Build history of the part. All positions in model axes, mm. A direction names the side the tool comes from. Round coordinates to 2 decimals unless told otherwise and drop trailing zeros. Write each loop counter-clockwise with the first axis right and the second up, starting at its lowest first coordinate (ties: lowest second). Pieces come first, ordered by that corner, then holes.
Autodesk Inventor part; units mm, degrees
ref_plane "YZ Plane" through (0, 0, 0) normal (1, 0, 0) x (0, 1, 0)
ref_plane "XZ Plane" through (0, 0, 0) normal (0, 1, 0) x (-1, 0, 0)
ref_plane "XY Plane" through (0, 0, 0) normal (0, 0, 1) x (1, 0, 0)
sketch "Sketch2" plane through (0, 0, 0) normal (0, 0, 1) x (1, 0, 0)
  line L0 (-10.8368, 23.5104) -> (-10.8368, -29.6906) construction
  line L1 (-37.8996, -2.6413) -> (16.2259, -2.6413) construction
  circle A0 centre (-28.9216, 37.4694) radius 2.4892
  circle A1 centre (7.248, 37.4694) radius 2.4892
  circle A2 centre (-28.9216, -20.4172) radius 2.4892
  circle A3 centre (7.248, -20.4172) radius 2.4892
  line L2 (-28.9216, 37.4694) -> (7.248, 37.4694) construction
  line L3 (7.248, 37.4694) -> (7.248, -20.4172) construction
  line L4 (7.248, -20.4172) -> (-28.9216, -20.4172) construction
  line L5 (-28.9216, -20.4172) -> (-28.9216, 37.4694) construction
  line L6 (-41.3549, 42.4478) -> (19.6813, 42.4478)
  line L7 (19.6813, 42.4478) -> (19.6813, -24.2272)
  line L8 (19.6813, -24.2272) -> (-41.3549, -24.2272)
  line L9 (-41.3549, -24.2272) -> (-41.3549, 42.4478)
  line L10 (-10.8368, 42.4478) -> (-10.8368, -24.2272) construction
  point P0 (0, 0)
  point P1 (-10.8368, -2.6413)
  dimension "d9" = 36.1696
  dimension "d10" = 57.8866
  dimension "d11" = 4.9784
  dimension "d12" = 61.0362
  dimension "d13" = 66.675
  dimension "d15" = 3.81
extrude "Extrusion1" add sketch "Sketch2" along normal blind 9.525
sketch "Sketch3" plane through (0, 0, 9.525) normal (0, 0, 1) x (1, 0, 0)
  line L0 (-41.3549, 34.1928) -> (19.6813, 34.1928)
  line L1 (19.6813, 34.1928) -> (19.6813, -16.6072)
  line L2 (19.6813, -16.6072) -> (-41.3549, -16.6072)
  line L3 (-41.3549, -16.6072) -> (-41.3549, 34.1928)
  line L4 (19.6813, -24.2272) -> (19.6813, 42.4478)
  line L5 (-41.3549, 42.4478) -> (-41.3549, -24.2272)
  line L6 (-41.3549, -24.2272) -> (19.6813, -24.2272)
  point P0 (0, 0)
  dimension "d18" = 50.8
  dimension "d20" = 7.62
extrude "Extrusion2" cut sketch "Sketch3" against normal blind 4.7498 contours L0 L1 L2 L3
chamfer "Chamfer1" distance 9.525 angle 45 4 edges at (19.6813, 42.4478, 4.7625) (-41.3549, 42.4478, 4.7625) (-41.3549, -24.2272, 4.7625) (19.6813, -24.2272, 4.7625)
fillet "Fillet1" radius 2.54 4 edges at (18.4113, 34.1928, 7.1501) (17.7763, -16.6072, 7.1501) (-39.4499, -16.6072, 7.1501) (-40.0849, 34.1928, 7.1501)
sketch "Sketch4" plane through (0, 0, 4.7752) normal (0, 0, 1) x (1, 0, 0)
  circle A0 centre (-10.8368, 7.2053) radius 14.2748
  line L0 (-41.3549, -14.7022) -> (-41.3549, 32.9228)
  line L1 (11.6442, -16.6072) -> (-33.3178, -16.6072)
  point P0 (0, 0)
  dimension "d27" = 30.5181
  dimension "d28" = 23.8125
  dimension "d29" = 28.5496
extrude "Extrusion3" cut sketch "Sketch4" against normal blind 4.7752
sketch "Sketch5" plane through (0, 0, 4.7752) normal (0, 0, 1) x (1, 0, 0)
  circle A0 centre (-10.8368, 7.2053) radius 14.2748
  circle A1 centre (-10.8368, 7.2053) radius 15.9766
  point P0 (0, 0)
  dimension "d32" = 31.9532
extrude "Extrusion4" cut sketch "Sketch5" against normal blind 1.6002
sketch "Sketch6" plane through (0, 0, 4.7752) normal (0, 0, 1) x (1, 0, 0)
  circle A0 centre (-10.8368, 7.2053) radius 14.2748
  circle A1 centre (-10.8368, 7.2053) radius 14.2748
  circle A2 centre (-10.8368, 7.2053) radius 23.8125 construction
  circle A3 centre (-34.6493, 7.2053) radius 2.4892
  point P0 (0, 0)
  dimension "d35" = 47.625
  dimension "d36" = 4.9784
extrude "Extrusion5" cut sketch "Sketch6" against normal through all contours A3
pattern_circular "Circular Pattern1" count 6 over 360 about axis through (-10.8368, 7.2053, 4.7752) along (0, 0, -1) of "Extrusion5"
sketch "Sketch7" plane through (0, 0, 4.7752) normal (0, 0, 1) x (1, 0, 0)
  circle A0 centre (-10.8368, 7.2053) radius 14.2748
  arc A1 (-5.4756, 27.2137) -> (-16.1981, 27.2137) centre (-10.8368, 7.2053) ccw
  arc A2 (-4.1608, 32.1206) -> (-17.5129, 32.1206) centre (-10.8368, 7.2053) ccw
  line L0 (-10.8368, 7.2053) -> (-10.8368, 32.9995) construction
  line L1 (-16.1981, 27.2137) -> (-17.5129, 32.1206)
  line L2 (-5.4756, 27.2137) -> (-4.1608, 32.1206)
  point P0 (0, 0)
  dimension "d42" = 5.08
extrude "Extrusion6" cut sketch "Sketch7" against normal through all contours A1 L1 A2 L2
pattern_circular "Circular Pattern2" count 6 over 360 about axis through (-10.8368, 7.2053, 4.7752) along (0, 0, -1) of "Extrusion6"
sketch "Sketch8" plane through (0, 0, 9.525) normal (0, 0, 1) x (1, 0, 0)
  line L0 (10.1563, 42.4478) -> (-31.8299, 42.4478)
  arc A0 (-25.4799, 42.4478) -> (3.8063, 42.4478) centre (-10.8368, 63.2021) ccw
  point P0 (0, 0)
  dimension "d49" = 6.35
  dimension "d50" = 6.35
  dimension "d51" = 25.4
extrude "Extrusion7" cut sketch "Sketch8" against normal through all
fillet "Fillet2" radius 2.54 2 edges at (-25.4799, 42.4478, 4.7625) (3.8063, 42.4478, 4.7625)
equation "\"d15\" = d14"
equation "\"d20\" = d19"
equation "\"d14\" = 3.81"
equation "\"d19\" = 2 * d14"
properties part number "Versa Chassis Bearing Block"
1) Wall check: L1, parallel to X at y = 7, z = 0.5; L2, parallel to X at y = -19, z = 7.75; L3, parallel to X at y = 14.5, z = 4.25. Give the ranges that are in metal, low to high.
Results:
L1: x = -41.35 to -37.13, -32.17 to -25.11, 3.44 to 10.49, 15.46 to 19.68
L2: x = -35.85 to -30.97, -26.88 to 5.2, 9.29 to 14.18
L3: x = -41.35 to -35.58, -30.22 to -25.05, 3.38 to 8.55, 13.9 to 19.68
2) Pin check, flat tips, straight feed: pin 1 Ø4.5 at (x, y) = (-22.74, 27.83) entering from +Z; pin 2 Ø1 at (x, z) = (-17.5, 5.5) entering from +Y; pin 3 Ø6.5 at (x, y) = (-22.74, -13.42) entering from +Z (3 decimals); pin 4 Ø12 at (x, y) = (-21, -4.5) entering from +Z. Stop position of each tip, or through.
Results:
pin 1: passes through
pin 2: stops at y = 38.83
pin 3: stops at z = 9.525
pin 4: stops at z = 4.78
3) Slice it at B-B (y = 20). Write the cut outline in (x, z) (3 decimals).
Results:
outline: (-41.355, 0) - (-33.234, 0) - (-33.234, 4.775) - (-41.355, 4.775) - close; (-27.127, 0) - (-17.167, 0) - (-17.167, 3.175) - (-20.405, 3.175) - (-20.405, 4.775) - (-27.127, 4.775) - close; (-4.507, 0) - (5.454, 0) - (5.454, 4.775) - (-1.269, 4.775) - (-1.269, 3.175) - (-4.507, 3.175) - close; (11.56, 0) - (19.681, 0) - (19.681, 4.775) - (11.56, 4.775) - close
4) Slice it at D-D (x = -2.5). Write the cut outline in (y, z) (3 decimals), plus the area to 3 significant figures.
Results:
outline: (-24.227, 0) - (-4.382, 0) - (-4.382, 3.175) - (-6.424, 3.175) - (-6.424, 4.775) - (-16.607, 4.775) - (-16.607, 9.525) - (-24.227, 9.525) - close; (18.793, 0) - (39.209, 0) - (39.209, 9.525) - (34.193, 9.525) - (34.193, 4.775) - (20.834, 4.775) - (20.834, 3.175) - (18.793, 3.175) - close
area: 246 mm2
5) Slice it at C-C (x = -30). Write the cut outline in (y, z) (3 decimals).
Results:
outline: (-24.227, 0) - (-22.661, 0) - (-22.661, 9.525) - (-24.227, 9.525) - close; (-18.174, 0) - (-10.061, 0) - (-10.061, 4.775) - (-16.607, 4.775) - (-16.607, 9.525) - (-18.174, 9.525) - close; (-0.659, 0) - (15.07, 0) - (15.07, 4.775) - (-0.659, 4.775) - close; (24.471, 0) - (35.226, 0) - (35.226, 9.525) - (34.193, 9.525) - (34.193, 4.775) - (24.471, 4.775) - close; (39.713, 0) - (42.448, 0) - (42.448, 9.525) - (39.713, 9.525) - close
6) Which spindle directions (+Z, -Z, +X, -X, +Y, -Y) get a long thin tool onto all of the face, cutting with end or side? Do faces 1 (the cylindrical face through (-10.91, -13.51, 2.42)), 2 (the flat face through (-11, -20, 9.525)), 3 (the cylindrical face through (-26.8, 7.9, 4)), 4 (the cylindrical face through (14.64, 35.8, 7.12)), 5 (the flat face through (-16.846, -15.222, 2.421)). Say none if no direction does.
Results:
face 1: +Z, -Z
face 2: +Z, +X, -X, +Y, -Y
face 3: +Z
face 4: +Z, +X
face 5: -Z
7) Mould opens along X. For faces 6 (the cylindrical face through (14, -18.2, 7.2)), 7 (the cylindrical face through (-36.28, 35.72, 7.12)), 8 (the cylindrical face through (11.55, 20.02, 2.42)) say: released by +X, released by -X, zero draft, split by the parting line, or undercut.
Results:
face 6: released by +X
face 7: released by -X
face 8: undercut
8) Slice it at A-A (z = 8.5). Write the cut outline in (x, y).
Results:
outline: (-35.75, 38.53) arc R2.54 ccw to (-33.95, 34.19) - (12.28, 34.19) arc R2.54 ccw to (14.08, 38.53) - (10.16, 42.45) - (4.59, 42.45) arc R2.54 ccw to (3.19, 42.03) arc R25.4 cw to (-24.86, 42.03) arc R2.54 ccw to (-26.26, 42.45) - (-31.83, 42.45) - close; (-35.11, -20.94) - (-31.83, -24.23) - (10.16, -24.23) - (13.44, -20.94) arc R2.54 ccw to (11.64, -16.61) - (-33.32, -16.61) arc R2.54 ccw to start; hole circle Ø4.98 at (-28.92, -20.42); hole circle Ø4.98 at (-28.92, 37.47); hole circle Ø4.98 at (7.25, -20.42); hole circle Ø4.98 at (7.25, 37.47)
